For this review, use the dimensioned drawing (mm, ordinates from the lowest corner) and the shaded views. Give positions to 0.01 mm unless a question says otherwise; leave off trailing zeros. Write each loop counter-clockwise with the first axis right and the second up, starting at its lowest first coordinate (ties: lowest second). Pieces come first, ordered by that corner, then holes. Notation, with made-up numbers: M 24,-39.75 L 35,-39.75 A13 cw 35,-28.75 Z; hole C 85.25,48 d6. An arc over 180 degrees is marked long. One line per item, written item: value. Start each with the question number.
Item 1: Consider section A-A, the plane z = 62.5. Write out the cut boundary in (x, y), and give its area (3 significant figures).
Item 2: Consider section B-B, the plane y = 104. Write out the cut boundary in (x, z), and give its area (3 significant figures).
Item 3: Consider section C-C, the plane y = 58.5. Write out the cut boundary in (x, z), and give its area (3 significant figures).
Item 4: To check wall thickness, follow probe 1 along Y at (x, z) = (5.25, 83.5); probe 2 along Z at (x, y) = (4.5, 50); probe 3 along Z at (x, y) = (1.5, 201.5). State the ranges of each line that lie inside material, in increasing order.
Item 5: Consider section D-D, the plane x = 2.25. Give the number of separate pieces and of enclosed holes in the cut face, and give its area (3 significant figures).
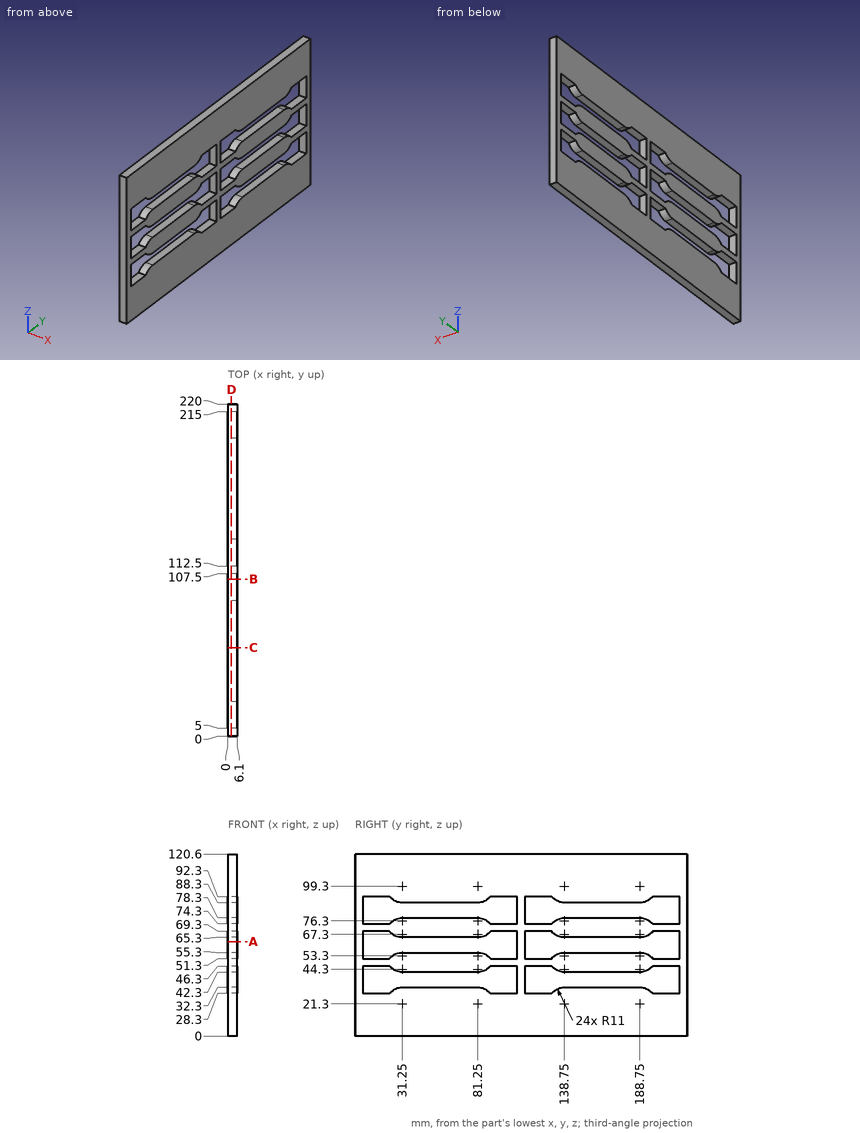
Model answer:
1. outline: M 0,0 L 6.1,0 L 6.1,5 L 0,5 Z; M 0,107.5 L 6.1,107.5 L 6.1,112.5 L 0,112.5 Z; M 0,215 L 6.1,215 L 6.1,220 L 0,220 Z
1. area: 91.5 mm2
2. outline: M 0,0 L 6.1,0 L 6.1,28.3 L 0,28.3 Z; M 0,46.3 L 6.1,46.3 L 6.1,51.3 L 0,51.3 Z; M 0,69.3 L 6.1,69.3 L 6.1,74.3 L 0,74.3 Z; M 0,92.3 L 6.1,92.3 L 6.1,120.6 L 0,120.6 Z
2. area: 406 mm2
3. outline: M 0,0 L 6.1,0 L 6.1,32.3 L 0,32.3 Z; M 0,42.3 L 6.1,42.3 L 6.1,55.3 L 0,55.3 Z; M 0,65.3 L 6.1,65.3 L 6.1,78.3 L 0,78.3 Z; M 0,88.3 L 6.1,88.3 L 6.1,120.6 L 0,120.6 Z
3. area: 553 mm2
4. probe 1: y = 0 to 5, 107.5 to 112.5, 215 to 220
4. probe 2: z = 0 to 32.3, 42.3 to 55.3, 65.3 to 78.3, 88.3 to 120.6
4. probe 3: z = 0 to 28.3, 46.3 to 51.3, 69.3 to 74.3, 92.3 to 120.6
5. separate pieces: 1
5. enclosed holes: 6
5. area: 18,400 mm2
